from build123d import *

# Parameters (mm, degrees)
F1_DEPTH    = 8.89
F3_DEPTH    = 7.62
F4_T1_DEPTH = 47.8505725861
F4_T3_DEPTH = 113.1511068404
F4_T6_ANGLE = 90
F4_T8_ANGLE = 90
F5_R        = 5.08
F6_R        = 3.81
F7_R        = 2.54


# Not quite as in the source:
# - a fillet or chamfer that OpenCascade refuses, or shapes differently, is made with other operations: its cross-section is extruded or revolved along the edge and cut away or added


with BuildPart() as f1:
    # F0 (on Top) → F1 (new body)
    with BuildSketch(Plane.XY):
        with BuildLine():
            Line((22.7506106496, 59.7472505152), (-90.4004961908, 59.7472505152))
            ThreePointArc((-90.4004961908, 59.7472505152), (-108.3610084329, 52.3077627574), (-115.8004961908, 34.3472505152))
            Line((-115.8004961908, 34.3472505152), (-115.8004961908, -13.5033220708))
            ThreePointArc((-115.8004961908, -13.5033220708), (-113.9406242513, -17.9934501314), (-109.4504961908, -19.8533220708))
            Line((-109.4504961908, -19.8533220708), (41.8006106496, -19.8533220708))
            ThreePointArc((41.8006106496, -19.8533220708), (46.2907387101, -17.9934501314), (48.1506106496, -13.5033220708))
            Line((48.1506106496, -13.5033220708), (48.1506106496, 34.3472505152))
            ThreePointArc((48.1506106496, 34.3472505152), (40.7111228917, 52.3077627574), (22.7506106496, 59.7472505152))
        make_face()
    extrude(amount=F1_DEPTH)

    # F2 (on face) → F3 (join)
    with BuildSketch(Plane.XY.offset(8.89)):
        with BuildLine():
            ThreePointArc((41.8006106496, -19.8533220708), (46.2907387101, -17.9934501314), (48.1506106496, -13.5033220708))
            Line((48.1506106496, -13.5033220708), (22.7506106496, -13.5033220708))
            Line((22.7506106496, -13.5033220708), (22.7506106496, -19.8533220708))
            Line((22.7506106496, -19.8533220708), (41.8006106496, -19.8533220708))
        make_face()
        with BuildLine():
            Line((-90.4004961908, -13.5033220708), (-115.8004961908, -13.5033220708))
            ThreePointArc((-115.8004961908, -13.5033220708), (-113.9406242513, -17.9934501314), (-109.4504961908, -19.8533220708))
            Line((-109.4504961908, -19.8533220708), (-90.4004961908, -19.8533220708))
            Line((-90.4004961908, -19.8533220708), (-90.4004961908, -13.5033220708))
        make_face()
    extrude(amount=F3_DEPTH)

    # F4: fillet of radius 2.54 on 1 edges, made by hand

    # F4_s2 → F4_t1 (cut)
    with BuildSketch(Plane.XZ.offset(-34.3472505152)):
        with BuildLine():
            ThreePointArc((45.6106106496, 8.89), (47.4066618738, 8.1460512242), (48.1506106496, 6.35))
            Line((48.1506106496, 6.35), (48.1506106496, 8.89))
            Line((48.1506106496, 8.89), (45.6106106496, 8.89))
        make_face()
        with BuildLine():
            ThreePointArc((-113.2604961908, 8.89), (-115.056547415, 8.1460512242), (-115.8004961908, 6.35))
            Line((-115.8004961908, 6.35), (-115.8004961908, 8.89))
            Line((-115.8004961908, 8.89), (-113.2604961908, 8.89))
        make_face()
    extrude(amount=F4_T1_DEPTH, mode=Mode.SUBTRACT)

    # F4_s4 → F4_t3 (cut)
    with BuildSketch(Plane.YZ.offset(-90.4004961908)):
        with BuildLine():
            ThreePointArc((57.2072505152, 8.89), (59.0033017394, 8.1460512242), (59.7472505152, 6.35))
            Line((59.7472505152, 6.35), (59.7472505152, 8.89))
            Line((59.7472505152, 8.89), (57.2072505152, 8.89))
        make_face()
    extrude(amount=F4_T3_DEPTH, mode=Mode.SUBTRACT)

    # F4_s5 → F4_t6 (revolve, cut)
    with BuildSketch(Plane.XZ.offset(-34.3472505152)):
        with BuildLine():
            ThreePointArc((48.1506106496, 6.35), (47.4066618738, 8.1460512242), (45.6106106496, 8.89))
            Line((45.6106106496, 8.89), (48.1506106496, 8.89))
            Line((48.1506106496, 8.89), (48.1506106496, 6.35))
        make_face()
    revolve(axis=Axis((22.7506106496, 34.3472505152, 8.89), (0, 0, 1)), revolution_arc=F4_T6_ANGLE, mode=Mode.SUBTRACT)

    # F4_s7 → F4_t8 (revolve, cut)
    with BuildSketch(Plane.YZ.offset(-90.4004961908)):
        with BuildLine():
            ThreePointArc((57.2072505152, 8.89), (59.0033017394, 8.1460512242), (59.7472505152, 6.35))
            Line((59.7472505152, 6.35), (59.7472505152, 8.89))
            Line((59.7472505152, 8.89), (57.2072505152, 8.89))
        make_face()
    revolve(axis=Axis((-90.4004961908, 34.3472505152, 8.89), (0, 0, 1)), revolution_arc=F4_T8_ANGLE, mode=Mode.SUBTRACT)

    # F5
    f5_edges = [f1.edges().sort_by_distance(p)[0] for p in [
        (-33.824943, 59.747251, 0),
    ]]
    fillet(f5_edges, radius=F5_R)

    # F6
    f6_edges = [f1.edges().sort_by_distance(p)[0] for p in [
        (35.450611, -13.503322, 16.51),
        (-103.100496, -13.503322, 16.51),
    ]]
    fillet(f6_edges, radius=F6_R)

    # F7
    f7_edges = [f1.edges().sort_by_distance(p)[0] for p in [
        (-90.400496, -19.853322, 12.7),
        (-33.824943, -19.853322, 8.89),
        (22.750611, -19.853322, 12.7),
    ]]
    fillet(f7_edges, radius=F7_R)


solid = f1.part
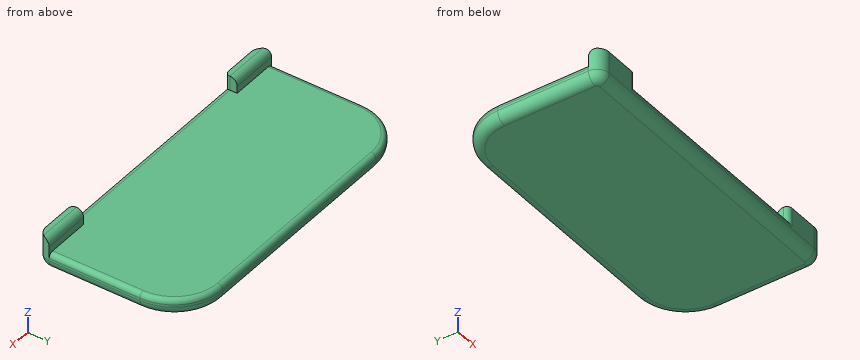
Read the model definition and answer for the solid it produces. Units are mm, in the model's axes. Round coordinates to 2 decimals unless told otherwise and drop trailing zeros. Loops run counter-clockwise (first coordinate to the right, second up) from the corner with the lowest first, then second, coordinate; pieces in that order, holes last.
Q1. Section A-A on z = 10.5 is taken. Write down the section's boundary in (x, y), and give its area (3 significant figures).
Q2. Consider probe 1 along X at (y, z) = (22.5, 6.5); probe 2 along Z at (x, y) = (-19.5, 23); probe 3 along X at (y, z) = (27, 1.75). Determine where each line is inside the solid, lowest interval first.
Q3. Section B-B on x = -10 is taken. Write down the section's boundary in (y, z), and give its area (3 significant figures).
Q4. Each of these flat-tipped pins is pushed along its axis until it touches: pin 1 (3 mm diameter, centred on x = -101.5, z = 9, fed in from +Y); pin 2 (8 mm diameter, centred on x = -5.5, y = -2, fed in from +Z); pin 3 (1.1 mm diameter, centred on y = -16.5, z = 12, fed in from -X). Where does it stop, or does it pass through?
Q5. Section C-C on y = 23.5 is taken. Write down the section's boundary in (x, z), and give its area (3 significant figures).
Output:
1. outline: (-115.8, -13.5) arc R6.35 ccw to (-109.45, -19.85) - (-92.94, -19.85) arc R2.54 ccw to (-90.4, -17.31) - (-90.4, -13.5) - close; (22.75, -17.31) arc R2.54 ccw to (25.29, -19.85) - (41.8, -19.85) arc R6.35 ccw to (48.15, -13.5) - (22.75, -13.5) - close
1. area: 303 mm2
2. probe 1: x = -115.8 to 48.15
2. probe 2: z = 0 to 8.89
2. probe 3: x = -114.56 to 46.91
3. outline: (-19.85, 5.08) arc R5.08 ccw to (-14.77, 0) - (54.67, 0) arc R5.08 ccw to (59.75, 5.08) - (59.75, 6.35) arc R2.54 ccw to (57.21, 8.89) - (-17.31, 8.89) arc R2.54 ccw to (-19.85, 6.35) - close
3. area: 694 mm2
4. pin 1: stops at y = 57.12
4. pin 2: stops at z = 8.89
4. pin 3: stops at x = -115.31
5. outline: (-115.8, 5.08) arc R5.08 ccw to (-110.72, 0) - (43.07, 0) arc R5.08 ccw to (48.15, 5.08) - (48.15, 6.35) arc R2.54 ccw to (45.61, 8.89) - (-113.26, 8.89) arc R2.54 ccw to (-115.8, 6.35) - close
5. area: 1,440 mm2
